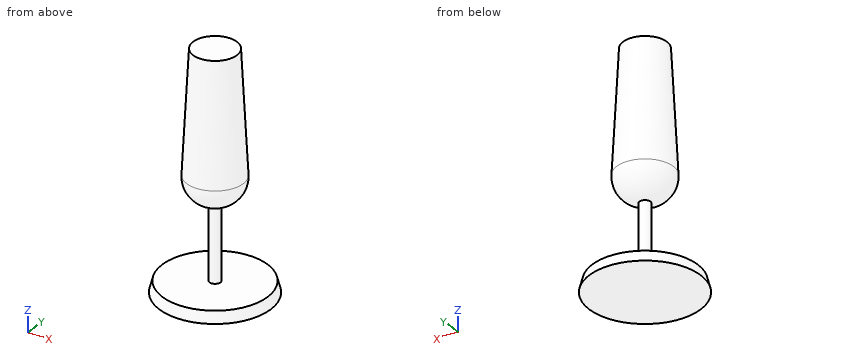
from build123d import *

# Parameters (mm, degrees)
F0_R     = 15
F1_DEPTH = 3
F1_TAPER = 15
F2_R     = 1.5
F3_DEPTH = 20
F4_R     = 8
F5_DEPTH = 40
F5_TAPER = 3


# Not quite as in the source:
# - a fillet or chamfer that OpenCascade refuses, or shapes differently, is made with other operations: its cross-section is extruded or revolved along the edge and cut away or added


with BuildPart() as f1:
    # F0 (on Top) → F1 (new body)
    with BuildSketch(Plane.XY):
        Circle(F0_R)
    extrude(amount=F1_DEPTH, taper=F1_TAPER)

    # F2 (on face) → F3 (join)
    with BuildSketch(Plane.XY.offset(3)):
        Circle(F2_R)
    extrude(amount=F3_DEPTH)

    # F4 (on face) → F5 (join)
    with BuildSketch(Plane.XY.offset(23)):
        Circle(F4_R)
    extrude(amount=F5_DEPTH, taper=F5_TAPER)

    # F6: fillet of radius 7 on 1 edges, made by hand

    # F6_s1 → F6_t2 (revolve, cut)
    with BuildSketch(Plane.XZ):
        with BuildLine():
            ThreePointArc((1.5, 23), (5.9953541002, 25.4536811979), (7.6168139169, 30.3116260276))
            Line((7.6168139169, 30.3116260276), (8, 23))
            Line((8, 23), (1.5, 23))
        make_face()
    revolve(axis=Axis((0, 0, 23), (0, 0, -1)), mode=Mode.SUBTRACT)


solid = f1.part
Source: CAD feature listing. Evaluate the final solid. Frame: model axes, mm. Coordinates: 2 decimals unless noted, no trailing zeros. Order: outer loops, then holes, each group sorted by start corner. A loop starts at its lowest first (then second) coordinate and runs counter-clockwise, first axis right, second up. Notation, with made-up numbers: M 6.25,-14.5 L 26.25,-14.5 A9 cw 26.25,-4.5 Z; hole C -19.5,-18 d5. An arc over 180 degrees is marked long. Write each question's results on one line, items separated by ' | '. Start each with the question number.
1. Pin query (flat end, axial travel): pin 1 (12 mm diameter, centred on y = -7.5, z = 23, fed in from +X); pin 2 (8 mm diameter, centred on x = 4.5, z = 29, fed in from -Y); pin 3 (12 mm diameter, centred on y = 0.5, z = 17.5, fed in from +X). Return the tip coordinate at first contact, or that it passes through.
2. Section A-A, the plane z = 9.5. Return the cut outline in (x, y).
3. Section B-B, the plane z = 33.5. Return the cut outline in (x, y).
4. Material intervals for L1, parallel to Z at x = -3.5, y = 1.5; L2, parallel to Z at x = 4, y = 2.5; L3, parallel to Z at x = -1.5, y = 9, sorted ascending.
Solution:
1) pin 1: x = 6.29 | pin 2: y = -7.6 | pin 3: x = 3.34
2) outline: C 0,0 d3
3) outline: C 0,0 d14.9
4) L1: 0 to 3, 23.71 to 63 | L2: 0 to 3, 24.26 to 63 | L3: 0 to 3
